Check sheet for the modelled part. Datum: model origin and axes. Units: mm. Face numbers are marked on the shaded views. A direction names the side the tool comes from. Round coordinates to 2 decimals unless told otherwise and drop trailing zeros. Loops run counter-clockwise (first coordinate to the right, second up) from the corner with the lowest first, then second, coordinate; pieces in that order, holes last. Notation, with made-up numbers: (87, -31) - (133, -31) arc R24 ccw to (133, -17) - close; hole circle Ø7 at (-10.75, 31). An arc over 180 degrees is marked (long way). Answer in a Markdown table with one row per item. Add a question column.
(1) Access from +Z, -Z, +X, -X, +Y, -Y to the whole of each face (thin tool, end or side, straight path). Record for the marked faces 1 and 2.
(2) Cross-section at D-D on y = 167. Enter the section's corners in (x, z), then the cut area to 3 significant figures.
(3) Cross-section at B-B on z = 121.5. Enter the section's corners in (x, y), then the cut area to 3 significant figures.
(4) Thickness scan on line 1 along Y through (x, z) = (45, 11); line 2 along Y through (x, z) = (122, 45.5). Record the ranges inside material, lowest first.
(5) Mould release check, pull along Y, two halves, no side actions. Record for the marked faces 3, 4, 5 and 6: +Y half, -Y half, draft (parallel to the pull), parting line (faces both ways), or undercut.
(6) Gauge pin test, flat ends, axial feed: pin 1 (1 mm diameter, centred on x = 111.5, y = 46.5, fed in from +Z); pin 2 (17.5 mm diameter, centred on x = 137.5, y = 45.5, fed in from +Z). Record the tip position at first contact, or that the pin passes through.
(7) Cross-section at A-A on y = 45. Enter the section's corners in (x, z), then the cut area to 3 significant figures.
Autodesk Fusion 360 part; units mm, degrees
sketch "Sketch1" plane through (0, 0, 0) normal (0, 0, 1) x (1, 0, 0)
  line L0 (0, 0) -> (180, 0)
  line L1 (180, 0) -> (180, 180)
  line L2 (180, 180) -> (0, 180)
  line L3 (0, 180) -> (0, 0)
  line L4 (-10, -10) -> (190, -10)
  line L5 (190, -10) -> (190, 190)
  line L6 (190, 190) -> (-10, 190)
  line L7 (-10, 190) -> (-10, -10)
  circle A0 centre (45, 45) radius 17.5
  circle A1 centre (45, 135) radius 17.5
  circle A2 centre (135, 135) radius 17.5
  circle A3 centre (135, 45) radius 17.5
  dimension "d1" = 180
  dimension "d2" = 180
  dimension "d3" = 35
  dimension "d4" = 35
  dimension "d5" = 45
  dimension "d6" = 45
  dimension "d7" = 45
  dimension "d8" = 45
  dimension "d9" = 35
  dimension "d10" = 45
  dimension "d11" = 45
  dimension "d12" = 35
  dimension "d13" = 45
  dimension "d14" = 45
extrude "Extrude1" add sketch "Sketch1" along normal blind 140 contours L4 L5 L6 L7
extrude "Extrude2" add sketch "Sketch1" against normal blind 30 contours L0 L1 L2 L3 | L4 L5 L6 L7 | A0 | A1 | A2 | A3
extrude "Extrude3" add sketch "Sketch1" along normal blind 30 contours L0 L1 L2 L3
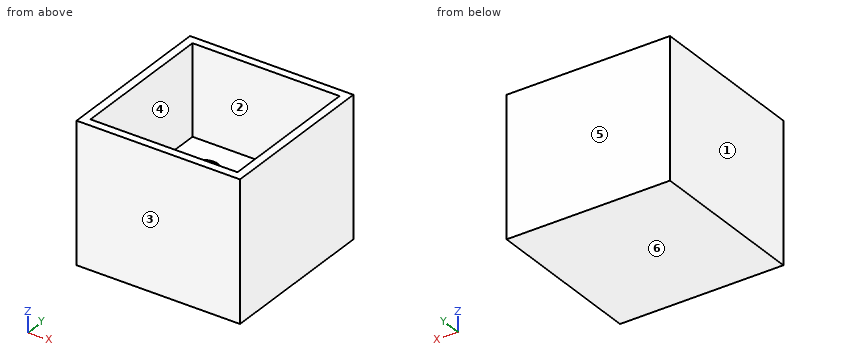
Answers:
| question | item | result |
|---|---|---|
| 1 | face 1 | +Z, -Z, -X, +Y, -Y |
| 1 | face 2 | +Z |
| 2 | outline | (-10, -30) - (190, -30) - (190, 140) - (180, 140) - (180, 30) - (0, 30) - (0, 140) - (-10, 140) - close |
| 2 | area | 14,200 mm^2 |
| 3 | outline | (-10, -10) - (190, -10) - (190, 190) - (-10, 190) - close; hole (0, 0) - (180, 0) - (180, 180) - (0, 180) - close |
| 3 | area | 7,600 mm^2 |
| 4 | line 1 | y = -10 to 27.5, 62.5 to 117.5, 152.5 to 190 |
| 4 | line 2 | y = -10 to 0, 180 to 190 |
| 5 | face 3 | -Y half |
| 5 | face 4 | undercut |
| 5 | face 5 | +Y half |
| 5 | face 6 | draft |
| 6 | pin 1 | stops at z = 30 |
| 6 | pin 2 | stops at z = 0 |
| 7 | outline | (-10, -30) - (190, -30) - (190, 140) - (180, 140) - (180, 30) - (152.5, 30) - (152.5, 0) - (117.5, 0) - (117.5, 30) - (62.5, 30) - (62.5, 0) - (27.5, 0) - (27.5, 30) - (0, 30) - (0, 140) - (-10, 140) - close |
| 7 | area | 12,100 mm^2 |
